For this review, take the finished solid that the model builds, in its own axes (mm). A direction names the side the tool comes from. Give positions to 0.01 mm unless a question says otherwise; leave off trailing zeros. Write each loop counter-clockwise with the first axis right and the second up, starting at its lowest first coordinate (ties: lowest second). Pieces come first, ordered by that corner, then holes. Notation, with made-up numbers: M 4.5,46 L 50.5,46 A31 ccw 50.5,82 Z; hole C 82.25,72.25 d3. An arc over 180 degrees is marked long. Use one line per item in the form item = value. Start each with the question number.
Q1. For probe 1 along X at (y, z) = (122, -1.75); probe 2 along X at (y, z) = (212, 9.55), list the stretches that pass through material, from the lowest coordinate up. Write a range as [from, to].
Q2. Tool access review of faces 4 (the flat face through (-9, 197, 0)), 5 (the flat face through (0, 197, 10)): name each direction out of +Z, -Z, +X, -X, +Y, -Y from which nothing blocks a thin tool from reaching the whole face with its end or side.
Q3. Consider section A-A on y = 261. Write out the cut boundary in (x, z), and give its area (3 significant figures).
Q4. Consider section B-B on z = 6. Write out the cut boundary in (x, y).
Q5. Clearance check with flat-ended pins moving along their axes: pin 1 Ø6 at (y, z) = (150, 0) entering from +X; pin 2 Ø2.5 at (y, z) = (390, 0) entering from -X. State where each tip first meets the part, or that it passes through.
Q6. Mouldability with a two-part tool opening along X and no side actions: class faces 1 (the flat face through (-0.8, 0, 9.6)), 2 (the flat face through (-10, 197, 0)), 3 (the flat face through (9, 197, 0)) as released by +X, released by -X, zero draft, split by the parting line, or undercut.
```python
from build123d import *

# Parameters (mm, degrees)
SKETCH1_W           = 20
SKETCH1_H           = 20
SKETCH1_W_2         = 18
SKETCH1_H_2         = 18
BOSS_EXTRUDE1_DEPTH = 400
SKETCH4_R           = 2.25
CUT_EXTRUDE1_DEPTH  = 401.62451248
SKETCH5_R           = 2.25
CUT_EXTRUDE2_DEPTH  = 401.62451248


with BuildPart() as part:
    # Sketch1 → Boss-Extrude1 (new body)
    with BuildSketch(Plane(origin=(0, 0, 0), x_dir=(1, 0, 0), z_dir=(0, 1, 0))):
        Rectangle(SKETCH1_W, SKETCH1_H)
        Rectangle(SKETCH1_W_2, SKETCH1_H_2, mode=Mode.SUBTRACT)
    extrude(amount=BOSS_EXTRUDE1_DEPTH)

    # Sketch4 → Cut-Extrude1 (cut, through all)
    with BuildSketch(Plane(origin=(0, 0, -10), x_dir=(-1, 0, 0), z_dir=(0, 0, -1))):
        with Locations((0, 20)):
            Circle(SKETCH4_R)
        with Locations((0, 40)):
            Circle(SKETCH4_R)
        with Locations((0, 60)):
            Circle(SKETCH4_R)
        with Locations((0, 80)):
            Circle(SKETCH4_R)
        with Locations((0, 188)):
            Circle(SKETCH4_R)
        with Locations(Location((0, 212, 0), (0, 0, 180))):
            Circle(SKETCH4_R)
    extrude(amount=-CUT_EXTRUDE1_DEPTH, mode=Mode.SUBTRACT)

    # Sketch5 → Cut-Extrude2 (cut, through all)
    with BuildSketch(Plane.ZY.offset(10)):
        with Locations((0, 188)):
            Circle(SKETCH5_R)
        with Locations((0, 212)):
            Circle(SKETCH5_R)
        with Locations((0, 110)):
            Circle(SKETCH5_R)
        with Locations((0, 130)):
            Circle(SKETCH5_R)
        with Locations((0, 150)):
            Circle(SKETCH5_R)
        with Locations(Location((0, 250, 0), (0, 0, 180))):
            Circle(SKETCH5_R)
        with Locations(Location((0, 290, 0), (0, 0, 180))):
            Circle(SKETCH5_R)
        with Locations(Location((0, 270, 0), (0, 0, 180))):
            Circle(SKETCH5_R)
        with Locations(Location((0, 390, 0), (0, 0, 180))):
            Circle(SKETCH5_R)
    extrude(amount=-CUT_EXTRUDE2_DEPTH, mode=Mode.SUBTRACT)


solid = part.part
```
Working result:
q1.probe_1 = [-10, -9], [9, 10]
q1.probe_2 = [-10, -2.25], [2.25, 10]
q2.face_4 = +Y, -Y
q2.face_5 = +Z, +X, -X, +Y, -Y
q3.outline = M -10,-10 L 10,-10 L 10,10 L -10,10 Z; hole M -9,-9 L 9,-9 L 9,9 L -9,9 Z
q3.area = 76.0 mm²
q4.outline = M -10,0 L -9,0 L -9,400 L -10,400 Z; M 9,0 L 10,0 L 10,400 L 9,400 Z
q5.pin_1 = 10
q5.pin_2 = through
q6.face_1 = zero draft
q6.face_2 = released by -X
q6.face_3 = undercut
